Source: three-view drawing plus pictorial views. Frame: mm from the lowest corner of the part. A direction names the side the tool comes from. Give positions to 0.01 mm unless a question says otherwise; leave off trailing zeros. Write each loop counter-clockwise with the first axis right and the second up, starting at its lowest first coordinate (ties: lowest second). Pieces come first, ordered by that corner, then holes.
Q1. Line query: L1, parallel to Z at x = 6, y = 1; L2, parallel to X at y = 0.3, z = 5; L3, parallel to X at y = 1.75, z = 2. Output: solid intervals per line, ascending.
Q2. Cut plane D-D on z = 7.5. Return the cut outline in (x, y).
Q3. Draft query along Z for the marked faces 1, 2, 3 and 4. Return one class per face: pulls with the +Z half, pulls with the -Z half, needs draft (parallel to the pull), parting line crosses it, or undercut.
Q4. Cut plane A-A on z = 5. Return the cut outline in (x, y), plus the area to 3 significant figures.
Q5. Cut plane C-C on x = 6.5. Return the cut outline in (y, z), plus the area to 3 significant figures.
Q6. Cut plane B-B on y = 6. Return the cut outline in (x, z).
Q7. Reachability of the marked faces 5 and 6 from +Z, -Z, +X, -X, +Y, -Y: full face, straight path, thin tool, end or side. Return the list, or none.
Q8. Pin query (flat end, axial travel): pin 1 (1.5 mm diameter, centred on y = 7.5, z = 7.5, fed in from +X); pin 2 (2 mm diameter, centred on x = 5.5, z = 6.5, fed in from +Y); pin 3 (1.8 mm diameter, centred on x = 6, z = 5, fed in from +Y). Return the tip coordinate at first contact, or that it passes through.
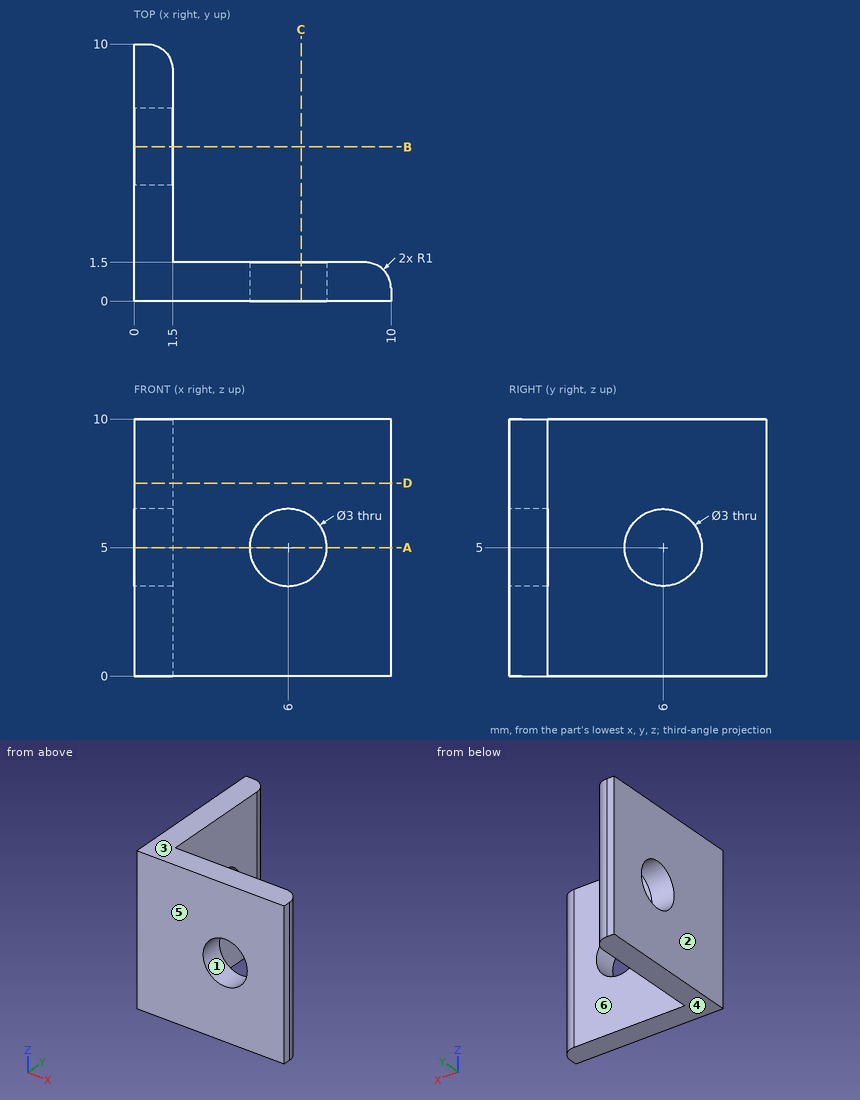
Data:
1. L1: z = 0 to 3.5, 6.5 to 10
1. L2: x = 0 to 4.5, 7.5 to 10
1. L3: x = 0 to 1.5
2. outline: (0, 0) - (10, 0) - (10, 0.5) arc R1 ccw to (9, 1.5) - (1.5, 1.5) - (1.5, 9) arc R1 ccw to (0.5, 10) - (0, 10) - close
3. face 1: undercut
3. face 2: needs draft
3. face 3: pulls with the +Z half
3. face 4: pulls with the -Z half
4. outline: (0, 0) - (4.5, 0) - (4.5, 1.5) - (1.5, 1.5) - (1.5, 4.5) - (0, 4.5) - close; (0, 7.5) - (1.5, 7.5) - (1.5, 9) arc R1 ccw to (0.5, 10) - (0, 10) - close; (7.5, 0) - (10, 0) - (10, 0.5) arc R1 ccw to (9, 1.5) - (7.5, 1.5) - close
4. area: 18.3 mm2
5. outline: (0, 0) - (1.5, 0) - (1.5, 3.59) - (0, 3.59) - close; (0, 6.41) - (1.5, 6.41) - (1.5, 10) - (0, 10) - close
5. area: 10.8 mm2
6. outline: (0, 0) - (1.5, 0) - (1.5, 3.5) - (0, 3.5) - close; (0, 6.5) - (1.5, 6.5) - (1.5, 10) - (0, 10) - close
7. face 5: +Z, -Z, +X, -X, -Y
7. face 6: +Z, -Z, +X, +Y
8. pin 1: stops at x = 1.5
8. pin 2: stops at y = 1.5
8. pin 3: passes through
